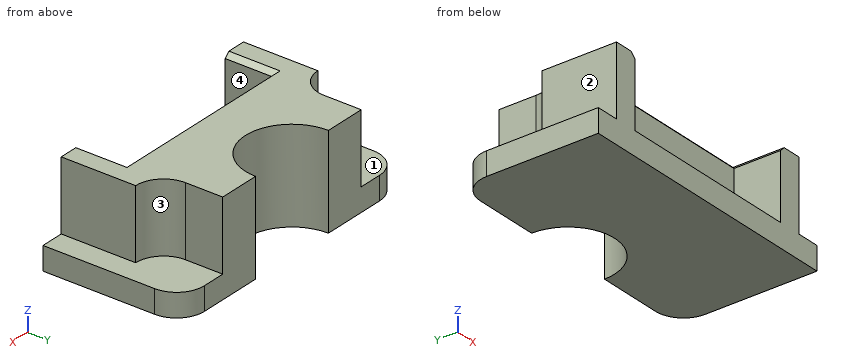
```python
from build123d import *

# Parameters (mm, degrees)
F0_W     = 76.2
F0_H     = 38.1
F1_DEPTH = 6.35
F3_DEPTH = 19.05
F5_DEPTH = 25.401
F6_W     = 7.62
F6_H     = 10.16
F7_DEPTH = 19.05
F8_SIZE  = 1.27
F9_R     = 7.62


with BuildPart() as f1:
    # F0 (on Top) → F1 (new body)
    with BuildSketch(Plane.XY):
        Rectangle(F0_W, F0_H)
    extrude(amount=F1_DEPTH)

    # F2 (on face) → F3 (join)
    with BuildSketch(Plane.XY.offset(6.35)):
        Polygon((31.75, 19.05), (-31.75, 19.05), (-31.75, -19.05), (-25.4, -19.05), (-25.4, -6.35), (25.4, -6.35), (25.4, -19.05), (31.75, -19.05), align=None)
    extrude(amount=F3_DEPTH)

    # F4 (on face) → F5 (cut, through all)
    with BuildSketch(Plane.XY.offset(25.4)):
        with BuildLine():
            ThreePointArc((-12.7, 19.05), (0, 6.35), (12.7, 19.05))
            Line((12.7, 19.05), (-12.7, 19.05))
        make_face()
    extrude(amount=-F5_DEPTH, mode=Mode.SUBTRACT)

    # F6 (on face) → F7 (cut, through all)
    with BuildSketch(Plane.XY.offset(25.4)):
        with BuildLine():
            Line((31.75, 1.27), (31.75, 8.89))
            Line((31.75, 8.89), (24.13, 8.89))
            ThreePointArc((24.13, 8.89), (26.3618463274, 3.5018463274), (31.75, 1.27))
        make_face()
        with Locations((27.94, 13.97)):
            Rectangle(F6_W, F6_H)
        with BuildLine():
            Line((-24.13, 8.89), (-24.13, 19.05))
            Line((-24.13, 19.05), (-31.75, 19.05))
            Line((-31.75, 19.05), (-31.75, 1.27))
            ThreePointArc((-31.75, 1.27), (-26.3618463274, 3.5018463274), (-24.13, 8.89))
        make_face()
    extrude(amount=-F7_DEPTH, mode=Mode.SUBTRACT)

    # F8
    f8_edges = [f1.edges().sort_by_distance(p)[0] for p in [
        (-25.4, -12.7, 25.4),
        (0, -6.35, 25.4),
        (25.4, -12.7, 25.4),
    ]]
    chamfer(f8_edges, length=F8_SIZE)

    # F9
    f9_edges = [f1.edges().sort_by_distance(p)[0] for p in [
        (-38.1, 19.05, 3.175),
        (38.1, 19.05, 3.175),
    ]]
    fillet(f9_edges, radius=F9_R)


solid = f1.part
```
Part model, mm, in its own coordinate system. Face numbers are marked on the shaded views. A direction names the side the tool comes from. Round coordinates to 2 decimals unless told otherwise and drop trailing zeros. Write each loop counter-clockwise with the first axis right and the second up, starting at its lowest first coordinate (ties: lowest second). Pieces come first, ordered by that corner, then holes. Notation, with made-up numbers: M 28,-8.5 L 39,-8.5 A17 ccw 39,-2.5 Z; hole C 24.25,-7 d6. An arc over 180 degrees is marked long. Answer as CSV lines item,"result". Start each with the question number.
1) Band-saw the part on C-C (z = 10). List the corners of the cut face in (x, y).
2) Which spindle directions (+Z, -Z, +X, -X, +Y, -Y) get a long thin tool onto all of the face, cutting with end or side? Do the marked faces 1, 2, 3 and 4. Say none if no direction does.
3) Band-saw the part on D-D (x = 0). List the corners of the cut face in (y, z).
4) Band-saw the part on A-A (x = -14). List the corners of the cut face in (y, z), then the cut area to 3 significant figures.
5) Band-saw the part on B-B (y = -3.5). List the corners of the cut face in (x, z), then the cut area to 3 significant figures.
6) Drill centre lines: L1, parallel to X at y = -14.5, z = 20; L2, parallel to Y at x = -22, z = 15.5; L3, parallel to Y at x = 0, z = 15.75. Where is each one in solid material? Low to high.
7) Drop flat-ended pins along their axis: pin 1 (5 mm diameter, centred on x = -14.5, y = 14.5, fed in from -Z); pin 2 (4 mm diameter, centred on y = -15.5, z = 16.5, fed in from +X); pin 3 (9.5 mm diameter, centred on y = -13.5, z = 16, fed in from -X); pin 4 (8 mm diameter, centred on x = -16, y = -12, fed in from +Z). Give the stop position or say it passes through.
Worked out:
1,outline,"M -31.75,-19.05 L -25.4,-19.05 L -25.4,-6.35 L 25.4,-6.35 L 25.4,-19.05 L 31.75,-19.05 L 31.75,1.27 A7.62 cw 24.13,8.89 L 24.13,19.05 L 12.7,19.05 A12.7 cw -12.7,19.05 L -24.13,19.05 L -24.13,8.89 A7.62 cw -31.75,1.27 Z"
2,face 1,"+Z, -X, +Y"
2,face 2,"+Z, -X, +Y, -Y"
2,face 3,"+Z, +X, +Y"
2,face 4,"+Z, -Y"
3,outline,"M -19.05,0 L 6.35,0 L 6.35,25.4 L -5.08,25.4 L -6.35,24.13 L -6.35,6.35 L -19.05,6.35 Z"
4,outline,"M -19.05,0 L 19.05,0 L 19.05,25.4 L -5.08,25.4 L -6.35,24.13 L -6.35,6.35 L -19.05,6.35 Z"
4,area,"725 mm²"
5,outline,"M -38.1,0 L 38.1,0 L 38.1,6.35 L 31.75,6.35 L 31.75,25.4 L -31.75,25.4 L -31.75,6.35 L -38.1,6.35 Z"
5,area,"1,690 mm²"
6,L1,"-31.75 to -25.4, 25.4 to 31.75"
6,L2,"-6.35 to 19.05"
6,L3,"-6.35 to 6.35"
7,pin 1,"z = 0"
7,pin 2,"x = 31.75"
7,pin 3,"x = -31.75"
7,pin 4,"z = 6.35"
